```python
from build123d import *

# Parameters (mm, degrees)
F1_DEPTH = 15
F2_R     = 1


with BuildPart() as f1:
    # F0 (on Right) → F1 (new body)
    with BuildSketch(Plane.YZ):
        Polygon((-4.25, 8.5), (-4.25, 0), (0, 0), (4.25, 0), (4.25, 8.5), (0, 11), align=None)
    extrude(amount=F1_DEPTH)

    # F2
    f2_edges = [f1.edges().sort_by_distance(p)[0] for p in [
        (7.5, -4.25, 8.5),
        (7.5, 0, 11),
        (7.5, 4.25, 8.5),
        (15, 2.125, 9.75),
        (15, -2.125, 9.75),
        (0, 2.125, 9.75),
        (0, -2.125, 9.75),
        (0, -4.25, 4.25),
        (0, 4.25, 4.25),
        (15, -4.25, 4.25),
        (15, 4.25, 4.25),
    ]]
    fillet(f2_edges, radius=F2_R)


solid = f1.part
```
Design review of the part built by this model. Coordinates are the model's own, in mm. Give positions to 0.01 mm unless a question says otherwise; leave off trailing zeros. Write each loop counter-clockwise with the first axis right and the second up, starting at its lowest first coordinate (ties: lowest second). Pieces come first, ordered by that corner, then holes.
(1) Clearance check with a flat-ended pin moving along its axis: pin 1 Ø5 at (x, y) = (8, -2) entering from +Z. State where the tip first meets the part, or that it passes through.
Checked values:
pin 1: stops at z = 10.84
(2) Add section A-A (x = 10). Give the boundary of the cut face in (y, z), and give its area (3 significant figures).
Checked values:
outline: (-4.25, 0) - (4.25, 0) - (4.25, 7.93) arc R1 ccw to (3.76, 8.79) - (0.51, 10.7) arc R1 ccw to (-0.51, 10.7) - (-3.76, 8.79) arc R1 ccw to (-4.25, 7.93) - close
area: 82.7 mm2
(3) Wall thickness on line 1 along Z through (x, y) = (2.25, 0.5); line 2 along Z through (x, y) = (6, 3.75); line 3 along Y through (x, z) = (7, 9.25) (3 decimals): over which ranges is each line inside the solid? List them lowest first.
Checked values:
line 1: z = 0 to 10.71
line 2: z = 0 to 8.79
line 3: y = -2.975 to 2.975
